Model file for the job. Use its own axes, mm. Face numbers are marked on the shaded views. A direction names the side the tool comes from. Coordinates: 2 decimals unless noted, no trailing zeros. Loops run counter-clockwise (first coordinate to the right, second up) from the corner with the lowest first, then second, coordinate; pieces in that order, holes last. Notation, with made-up numbers: (2, -11) -> (41, -11) arc R16 cw to (41, 18) -> close; hole circle Ø2 at (59, 77). An arc over 180 degrees is marked (long way). Use one line per item in the form item = value.
```python
from build123d import *

# Parameters (mm, degrees)
SKETCH004_W             = 35
SKETCH004_H             = 20
PAD001_DEPTH            = 20
POCKET003_DEPTH         = 100
SKETCH007_R             = 2.675
POCKET004_DEPTH         = 100
POCKET005_DEPTH         = 10
BODY001_PLACEMENT_ANGLE = 90


with BuildPart() as part:
    # Sketch004 → Pad001 (new body)
    with BuildSketch(Plane.XY):
        Rectangle(SKETCH004_W, SKETCH004_H)
    extrude(amount=PAD001_DEPTH)

    # Sketch005 (on Face2 of Pad001) → Pocket003 (cut)
    with BuildSketch(Plane.YZ.offset(17.5)):
        Polygon((2.352702, 14.075), (-2.352702, 14.075), (-4.705405, 10), (-2.352702, 5.925), (2.352702, 5.925), (4.705405, 10), align=None)
    extrude(amount=-POCKET003_DEPTH, mode=Mode.SUBTRACT)

    # Sketch007 (on Face5 of Pocket003) → Pocket004 (cut)
    with BuildSketch(Plane.XY.offset(20)):
        Circle(SKETCH007_R)
    extrude(amount=-POCKET004_DEPTH, mode=Mode.SUBTRACT)

    # Sketch008 (on Face4 of Pocket004) → Pocket005 (cut)
    with BuildSketch(Plane(origin=(0, 0, 0), x_dir=(1, 0, 0), z_dir=(0, 0, -1))):
        Polygon((4.705405, 0), (2.352702, 4.075), (-2.352702, 4.075), (-4.705405, 0), (-2.352702, -4.075), (2.352702, -4.075), align=None)
    extrude(amount=-POCKET005_DEPTH, mode=Mode.SUBTRACT)


with BuildPart() as part_1:
    # Body001 placement: moved
    add(part.part.rotate(Axis((0, 0, 0), (0, 0, 1)), BODY001_PLACEMENT_ANGLE))


solid = part_1.part
```
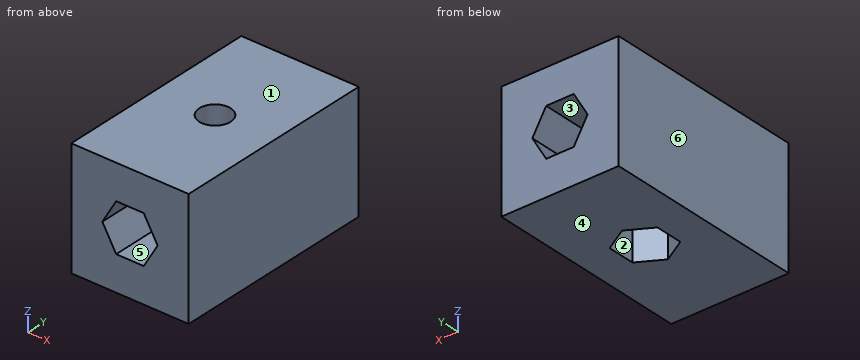
Q1. Mould opens along X. For the marked faces 4, 5 and 6 say: released by +X, released by -X, zero draft, split by the parting line, or undercut.
Result:
face_4 = zero draft
face_5 = undercut
face_6 = released by -X
Q2. Band-saw the part on A-A, the plane z = 5.5. Write the cut outline in (x, y) (3 decimals), and give its area (3 significant figures).
Result:
outline = (-10, -17.5) -> (10, -17.5) -> (10, 17.5) -> (-10, 17.5) -> close; hole (-4.075, -2.353) -> (0, -4.705) -> (4.075, -2.353) -> (4.075, 2.353) -> (0, 4.705) -> (-4.075, 2.353) -> close
area = 642 mm2
Q3. Which spindle directions (+Z, -Z, +X, -X, +Y, -Y) get a long thin tool onto all of the face, cutting with end or side? Do the marked faces 1, 2 and 3. Say none if no direction does.
Result:
face_1 = +Z, +X, -X, +Y, -Y
face_2 = -Z
face_3 = +Y, -Y
Q4. Band-saw the part on C-C, the plane x = -3.25. Write the cut outline in (y, z), and give its area (3 significant figures).
Result:
outline = (-17.5, 0) -> (-2.83, 0) -> (-2.83, 7.48) -> (-17.5, 7.48) -> close; (-17.5, 12.52) -> (17.5, 12.52) -> (17.5, 20) -> (-17.5, 20) -> close; (2.83, 0) -> (17.5, 0) -> (17.5, 7.48) -> (2.83, 7.48) -> close
area = 481 mm2
Q5. Wall check: line 1 along Y through (x, z) = (0.5, 16.25); line 2 along X through (y, z) = (0, 18.75) (3 decimals); line 3 along Z through (x, y) = (-2.5, -6.5). Give the ranges that are in metal, low to high.
Result:
line_1 = -17.5 to -2.63, 2.63 to 17.5
line_2 = -10 to -2.675, 2.675 to 10
line_3 = 0 to 6.18, 13.82 to 20
Q6. Pin check, flat tips, straight feed: pin 1 Ø4 at (x, y) = (-6, -2.5) entering from -Z; pin 2 Ø5 at (x, y) = (0, 0) entering from -Z. Stop position of each tip, or through.
Result:
pin_1 = 0
pin_2 = through
Q7. Band-saw the part on D-D, the plane y = 0. Write the cut outline in (x, z) (3 decimals), and give its area (3 significant figures).
Result:
outline = (-10, 0) -> (-4.075, 0) -> (-4.075, 8.908) -> (-4.705, 10) -> (-2.675, 13.517) -> (-2.675, 20) -> (-10, 20) -> close; (2.675, 13.517) -> (4.705, 10) -> (4.075, 8.908) -> (4.075, 0) -> (10, 0) -> (10, 20) -> (2.675, 20) -> close
area = 257 mm2
Q8. Band-saw the part on B-B, the plane y = -11. Write the cut outline in (x, z) (3 decimals).
Result:
outline = (-10, 0) -> (10, 0) -> (10, 20) -> (-10, 20) -> close; hole (-4.705, 10) -> (-2.353, 5.925) -> (2.353, 5.925) -> (4.705, 10) -> (2.353, 14.075) -> (-2.353, 14.075) -> close
